The model under review builds one solid part; all positions refer to its coordinate system, in mm. Coordinates: 2 decimals unless noted, no trailing zeros. Order: outer loops, then holes, each group sorted by start corner. A loop starts at its lowest first (then second) coordinate and runs counter-clockwise, first axis right, second up. Notation, with made-up numbers: (51.5, 26.25) -> (72.5, 26.25) arc R18 ccw to (72.5, 38.25) -> close; hole circle Ø2 at (10.25, -11). An arc over 180 degrees is marked (long way). Use one line per item in the form item = value.
from build123d import *

# Parameters (mm, degrees)
SKETCH1_R                     = 100
SKETCH1_R_2                   = 30
BOSS_EXTRUDE1_DEPTH           = 2.5
SKETCH2_R                     = 1.8
BOSS_EXTRUDE2_DEPTH           = 2
BOSS_EXTRUDE2_DRAFT           = -2
BOSS_EXTRUDE2_PROFILE_2_DEPTH = 2
BOSS_EXTRUDE2_PROFILE_2_DRAFT = -2
BOSS_EXTRUDE2_PROFILE_3_DEPTH = 2
BOSS_EXTRUDE2_PROFILE_3_DRAFT = -2
BOSS_EXTRUDE2_PROFILE_4_DEPTH = 2
BOSS_EXTRUDE2_PROFILE_4_DRAFT = -2
SKETCH5_W                     = 43
SKETCH5_H                     = 30
BOSS_EXTRUDE4_DEPTH           = 2.35
CUT_EXTRUDE1_DEPTH            = 142.492932686
CUT_EXTRUDE1_DEPTH_BACK       = 142.492932686
SKETCH4_R                     = 2
CUT_EXTRUDE2_DEPTH            = 142.492932686


with BuildPart() as part:
    # Sketch1 → Boss-Extrude1 (new body)
    with BuildSketch(Plane(origin=(0, 0, 0), x_dir=(1, 0, 0), z_dir=(0, 1, 0))):
        with Locations(Location((0, 0, 0), (0, 0, 270))):
            Circle(SKETCH1_R)
        with Locations(Location((0, 0, 0), (0, 0, 270))):
            Circle(SKETCH1_R_2, mode=Mode.SUBTRACT)
    extrude(amount=BOSS_EXTRUDE1_DEPTH)


with BuildPart() as boss_extrude2_tool:
    # Sketch2 → Boss-Extrude2 (with draft: the straight prism first)
    with BuildSketch(Plane(origin=(0, 2.5, 0), x_dir=(1, 0, 0), z_dir=(0, 1, 0))):
        with Locations((-32.75, 32.75)):
            Circle(SKETCH2_R)
    extrude(amount=BOSS_EXTRUDE2_DEPTH)
    # Boss-Extrude2: the draft: its side faces are tilted about the plane it starts from
    boss_extrude2_sides = [boss_extrude2_tool.faces().sort_by_distance(p)[0] for p in [
        (-34.55, 3.5, -32.75),
    ]]
    draft(boss_extrude2_sides, Plane(origin=(0, 2.5, 0), x_dir=(1, 0, 0), z_dir=(0, 1, 0)), BOSS_EXTRUDE2_DRAFT)


with BuildPart() as part_1:
    add(part.part)

    # Boss-Extrude2: add boss_extrude2_tool
    add(boss_extrude2_tool.part)


with BuildPart() as boss_extrude2_profile_2_tool:
    # Sketch2 → Boss-Extrude2 profile 2 (with draft: the straight prism first)
    with BuildSketch(Plane(origin=(0, 2.5, 0), x_dir=(1, 0, 0), z_dir=(0, 1, 0))):
        with Locations((-32.75, -32.75)):
            Circle(SKETCH2_R)
    extrude(amount=BOSS_EXTRUDE2_PROFILE_2_DEPTH)
    # Boss-Extrude2 profile 2: the draft: its side faces are tilted about the plane it starts from
    boss_extrude2_profile_2_sides = [boss_extrude2_profile_2_tool.faces().sort_by_distance(p)[0] for p in [
        (-34.55, 3.5, 32.75),
    ]]
    draft(boss_extrude2_profile_2_sides, Plane(origin=(0, 2.5, 0), x_dir=(1, 0, 0), z_dir=(0, 1, 0)), BOSS_EXTRUDE2_PROFILE_2_DRAFT)


with BuildPart() as part_2:
    add(part_1.part)

    # Boss-Extrude2 profile 2: add boss_extrude2_profile_2_tool
    add(boss_extrude2_profile_2_tool.part)


with BuildPart() as boss_extrude2_profile_3_tool:
    # Sketch2 → Boss-Extrude2 profile 3 (with draft: the straight prism first)
    with BuildSketch(Plane(origin=(0, 2.5, 0), x_dir=(1, 0, 0), z_dir=(0, 1, 0))):
        with Locations((32.75, -32.75)):
            Circle(SKETCH2_R)
    extrude(amount=BOSS_EXTRUDE2_PROFILE_3_DEPTH)
    # Boss-Extrude2 profile 3: the draft: its side faces are tilted about the plane it starts from
    boss_extrude2_profile_3_sides = [boss_extrude2_profile_3_tool.faces().sort_by_distance(p)[0] for p in [
        (30.95, 3.5, 32.75),
    ]]
    draft(boss_extrude2_profile_3_sides, Plane(origin=(0, 2.5, 0), x_dir=(1, 0, 0), z_dir=(0, 1, 0)), BOSS_EXTRUDE2_PROFILE_3_DRAFT)


with BuildPart() as part_3:
    add(part_2.part)

    # Boss-Extrude2 profile 3: add boss_extrude2_profile_3_tool
    add(boss_extrude2_profile_3_tool.part)


with BuildPart() as boss_extrude2_profile_4_tool:
    # Sketch2 → Boss-Extrude2 profile 4 (with draft: the straight prism first)
    with BuildSketch(Plane(origin=(0, 2.5, 0), x_dir=(1, 0, 0), z_dir=(0, 1, 0))):
        with Locations((32.75, 32.75)):
            Circle(SKETCH2_R)
    extrude(amount=BOSS_EXTRUDE2_PROFILE_4_DEPTH)
    # Boss-Extrude2 profile 4: the draft: its side faces are tilted about the plane it starts from
    boss_extrude2_profile_4_sides = [boss_extrude2_profile_4_tool.faces().sort_by_distance(p)[0] for p in [
        (30.95, 3.5, -32.75),
    ]]
    draft(boss_extrude2_profile_4_sides, Plane(origin=(0, 2.5, 0), x_dir=(1, 0, 0), z_dir=(0, 1, 0)), BOSS_EXTRUDE2_PROFILE_4_DRAFT)


with BuildPart() as part_4:
    add(part_3.part)

    # Boss-Extrude2 profile 4: add boss_extrude2_profile_4_tool
    add(boss_extrude2_profile_4_tool.part)

    # Sketch5 → Boss-Extrude4 (add)
    with BuildSketch(Plane.XZ):
        with Locations((0, -69.45)):
            Rectangle(SKETCH5_W, SKETCH5_H)
    extrude(amount=BOSS_EXTRUDE4_DEPTH)

    # Sketch4 → Cut-Extrude1 (cut, two sides: drawn at the far end of the back side and taken through both)
    with BuildSketch(Plane.XZ.offset(-CUT_EXTRUDE1_DEPTH_BACK)):
        with Locations(Location((-14.675074607, -69.517945059, 0), (0, 0, 270))):
            Circle(SKETCH4_R)
        with Locations(Location((14.675074607, -69.517945059, 0), (0, 0, 270))):
            Circle(SKETCH4_R)
    extrude(amount=CUT_EXTRUDE1_DEPTH + CUT_EXTRUDE1_DEPTH_BACK, mode=Mode.SUBTRACT)

    # Sketch6 → Cut-Extrude2 (cut, through all)
    with BuildSketch(Plane.XZ):
        with BuildLine():
            Line((48.863066456, -10.601921361), (30.5, -95.235235076))
            ThreePointArc((30.5, -95.235235076), (80.777472107, -58.949130613), (100, 0))
            ThreePointArc((100, 0), (-58.949130613, 80.777472107), (-30.5, -95.235235076))
            Line((-30.5, -95.235235076), (-48.863066456, -10.601921361))
            ThreePointArc((-48.863066456, -10.601921361), (-5.331354294, 49.714954102), (50, 0))
            ThreePointArc((50, 0), (49.714954102, -5.331354294), (48.863066456, -10.601921361))
        make_face()
    extrude(amount=-CUT_EXTRUDE2_DEPTH, mode=Mode.SUBTRACT)


solid = part_4.part
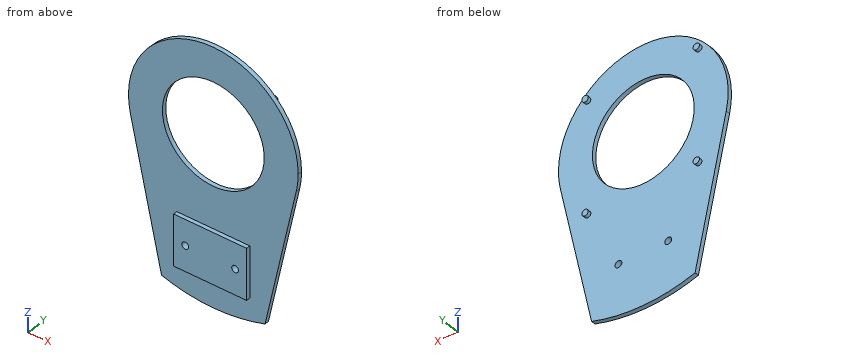
Item 1: To check wall thickness, follow L1, parallel to Z at x = 13.5, y = 1; L2, parallel to Y at x = -35, z = -65; L3, parallel to Z at x = 13, y = 0.5. State the ranges of each line that lie inside material, in increasing order. Write a range as from..to.
Results found:
L1 = -99.08..-71.14, -67.9..-26.79, 26.79..48.14
L2 = 0..2.5
L3 = -99.15..-70.61, -68.43..-27.04, 27.04..48.28
Item 2: We need section A-A (x = 0). Write out the cut boundary in (y, z), plus the area to 4 significant figures.
Results found:
outline = (-2.35, -84.45) -> (0, -84.45) -> (0, -100) -> (2.5, -100) -> (2.5, -30) -> (0, -30) -> (0, -54.45) -> (-2.35, -54.45) -> close; (0, 30) -> (2.5, 30) -> (2.5, 50) -> (0, 50) -> close
area = 295.5 mm²
Item 3: We need section C-C (x = -32.75). Write out the cut boundary in (y, z), plus the area to 3 significant figures.
Results found:
outline = (0, -84.87) -> (2.5, -84.87) -> (2.5, -34.55) -> (4.5, -34.62) -> (4.5, -30.88) -> (2.5, -30.95) -> (2.5, 30.95) -> (4.5, 30.88) -> (4.5, 34.62) -> (2.5, 34.55) -> (2.5, 37.78) -> (0, 37.78) -> close
area = 321 mm²
Item 4: We need section B-B (z = 3). Write out the cut boundary in (x, y), plus the area to 3 significant figures.
Results found:
outline = (-49.91, 0) -> (-29.85, 0) -> (-29.85, 2.5) -> (-49.91, 2.5) -> close; (29.85, 0) -> (49.91, 0) -> (49.91, 2.5) -> (29.85, 2.5) -> close
area = 100 mm²
Item 5: We need section D-D (z = -76.5). Write out the cut boundary in (x, y), plus the area to 3 significant figures.
Results found:
outline = (-34.57, 0) -> (-21.5, 0) -> (-21.5, -2.35) -> (21.5, -2.35) -> (21.5, 0) -> (34.57, 0) -> (34.57, 2.5) -> (-34.57, 2.5) -> close
area = 274 mm²
Item 6: Clearance check with flat-ended pins moving along their axes: pin 1 (4.5 mm diameter, centred on x = -14.68, z = -69.52, fed in from -Y); pin 2 (5 mm diameter, centred on x = 37, z = 28.5, fed in from +Y); pin 3 (2.5 mm diameter, centred on x = -4.5, y = -0.5, fed in from -Z); pin 4 (0.7 mm diameter, centred on y = -1, z = -76, fed in from -X). State where each tip first meets the part, or that it passes through.
Results found:
pin_1 = -2.35
pin_2 = 2.5
pin_3 = -99.94
pin_4 = -21.5
